CAD build for the part. Positions are in the model's coordinates, mm. A direction names the side the tool comes from. Round coordinates to 2 decimals unless told otherwise and drop trailing zeros. Order: outer loops, then holes, each group sorted by start corner. A loop starts at its lowest first (then second) coordinate and runs counter-clockwise, first axis right, second up. Notation, with made-up numbers: (-22, 37) - (-8, 37) arc R18 ccw to (-8, 46) - close; hole circle Ø1 at (65, -28). An arc over 180 degrees is marked (long way). Write item = value, one per line.
from build123d import *

# Parameters (mm, degrees)
BOSS_EXTRUDE1_DEPTH = 7
FILLET2_R           = 5
SKETCH2_W           = 170.284513749
SKETCH2_H           = 106.858227508
CUT_EXTRUDE1_DEPTH  = 2


with BuildPart() as part:
    # Sketch1 → Boss-Extrude1 (new body)
    with BuildSketch(Plane.XY):
        with BuildLine():
            Line((-176.117936118, 85.073710074), (43.882063882, 85.073710074))
            ThreePointArc((43.882063882, 85.073710074), (50.953131694, 82.144777886), (53.882063882, 75.073710074))
            Line((53.882063882, 75.073710074), (53.882063882, -73.926289926))
            ThreePointArc((53.882063882, -73.926289926), (50.953131694, -80.997357738), (43.882063882, -83.926289926))
            Line((43.882063882, -83.926289926), (-176.117936118, -83.926289926))
            ThreePointArc((-176.117936118, -83.926289926), (-183.18900393, -80.997357738), (-186.117936118, -73.926289926))
            Line((-186.117936118, -73.926289926), (-186.117936118, 75.073710074))
            ThreePointArc((-186.117936118, 75.073710074), (-183.18900393, 82.144777886), (-176.117936118, 85.073710074))
        make_face()
    extrude(amount=BOSS_EXTRUDE1_DEPTH)

    # Fillet2
    fillet2_edges = [part.edges().sort_by_distance(p)[0] for p in [
        (-183.18900393, -80.997357738, 7),
        (-66.117936118, -83.926289926, 7),
        (50.953131694, -80.997357738, 7),
        (53.882063882, 0.573710074, 7),
        (50.953131694, 82.144777886, 7),
        (-66.117936118, 85.073710074, 7),
        (-183.18900393, 82.144777886, 7),
        (-186.117936118, 0.573710074, 7),
    ]]
    fillet(fillet2_edges, radius=FILLET2_R)

    # Sketch2 → Cut-Extrude1 (cut, symmetric)
    with BuildSketch(Plane.XY.offset(3.5)):
        with Locations((-70.48620655, -6.89321053)):
            Rectangle(SKETCH2_W, SKETCH2_H)
    extrude(amount=CUT_EXTRUDE1_DEPTH, both=True, mode=Mode.SUBTRACT)


solid = part.part
(1) Probe line 1 along Z through (x, y) = (-70.5, -5.5); line 2 along Y through (x, z) = (-59, 2.5); line 3 along X through (y, z) = (-55, 1.75). List the from-to ranges inside material, lowest first.
Solved:
line_1 = 0 to 1.5, 5.5 to 7
line_2 = -83.9 to -60.32, 46.54 to 85.05
line_3 = -186.12 to -155.63, 14.66 to 53.88
(2) Band-saw the part on A-A on y = 39.5. List the corners of the cut face in (x, z).
Solved:
outline = (-186.12, 0) - (53.88, 0) - (53.88, 2) arc R5 ccw to (48.88, 7) - (-181.12, 7) arc R5 ccw to (-186.12, 2) - close; hole (-155.63, 1.5) - (14.66, 1.5) - (14.66, 5.5) - (-155.63, 5.5) - close
(3) Band-saw the part on B-B on x = -86. List the corners of the cut face in (y, z).
Solved:
outline = (-83.93, 0) - (85.07, 0) - (85.07, 2) arc R5 ccw to (80.07, 7) - (-78.93, 7) arc R5 ccw to (-83.93, 2) - close; hole (-60.32, 1.5) - (46.54, 1.5) - (46.54, 5.5) - (-60.32, 5.5) - close
(4) Pull direction Z, two halves, no side cores. Call faces 1 (the flat face through (-64, 2, 0)), 2 (the flat face through (-72, -6, 1.5)), 3 (the cylindrical face through (-184.69, 1.62, 5.5)): released by +Z, released by -Z, zero draft, split by the parting line, or undercut.
Solved:
face_1 = released by -Z
face_2 = undercut
face_3 = released by +Z
(5) Drop flat-ended pins along their axis: pin 1 (3 mm diameter, centred on x = -62.5, z = 4, fed in from +Y); pin 2 (1.2 mm diameter, centred on y = 2, z = 4, fed in from -X). Give the stop position or say it passes through.
Solved:
pin_1 = 85.05
pin_2 = -185.92
(6) Tool access for faces 4 (the cylindrical face through (52.456, -0.469, 5.496)), 5 (the flat face through (-72, -6, 5.5)): list every direction of +Z, -Z, +X, -X, +Y, -Y with a clear straight run to the whole face (end or side of a thin tool).
Solved:
face_4 = +Z, +X, +Y, -Y
face_5 = none
